Answer from the drawing. Dimensions are ordinates in mm from the lowest x, y and z of the part. A direction names the side the tool comes from. Coordinates: 2 decimals unless noted, no trailing zeros. Loops run counter-clockwise (first coordinate to the right, second up) from the corner with the lowest first, then second, coordinate; pieces in that order, holes last. Notation, with made-up numbers: (-6, 49) -> (47, 49) arc R14 ccw to (47, 57) -> close; hole circle Ø10 at (-20, 82.5). An arc over 180 degrees is marked (long way). Use a Markdown table: item, result.
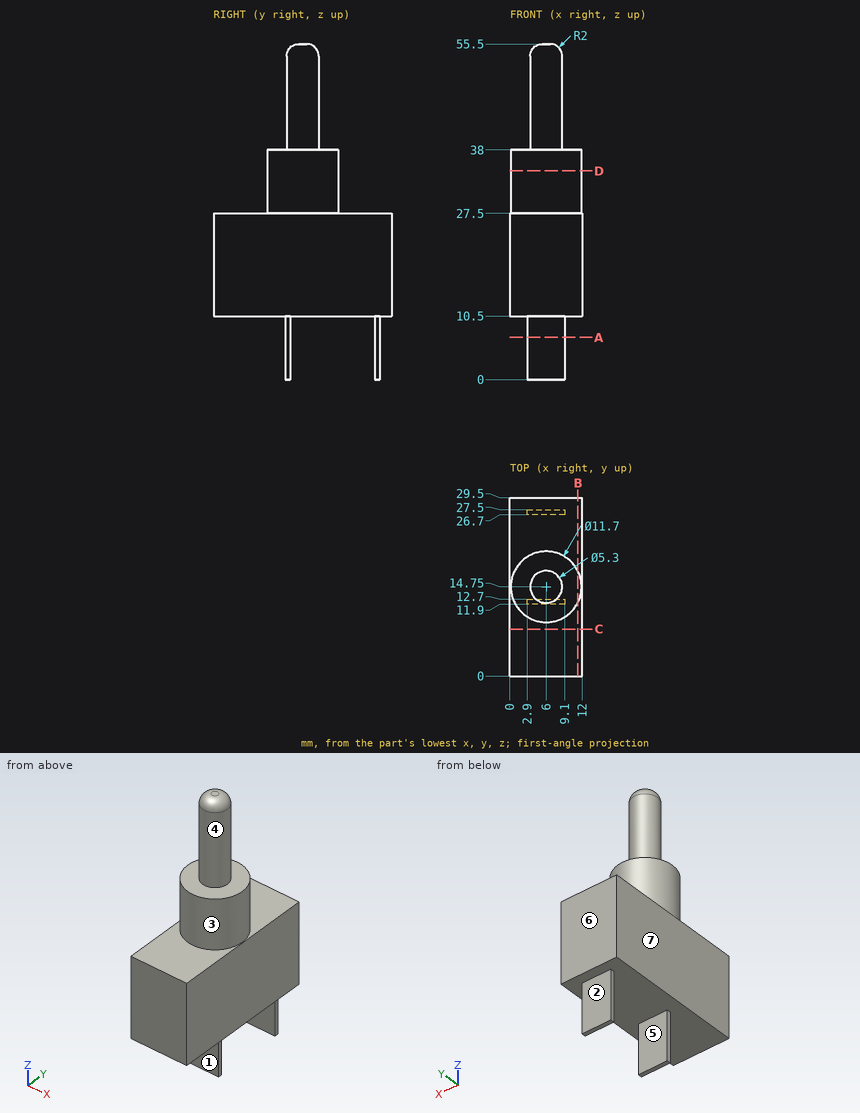
Q1. Consider line 1 (Y direction, x = 8.5, z = 6); line 2 (Z direction, x = 6.5, y = 19.25); line 3 (Z direction, x = 1.5, y = 10). Determine where each line is inside the solid, lowest interval first. Write a range as [from, to].
Solved:
| item | result |
|---|---|
| line 1 | [11.9, 12.7], [26.7, 27.5] |
| line 2 | [10.5, 38] |
| line 3 | [10.5, 27.5] |
Q2. Section B-B on x = 11.25 is taken. Determine the outline of the cut face in (y, z), and give its area (3 significant figures).
Solved:
| item | result |
|---|---|
| outline | (0, 10.5) -> (29.5, 10.5) -> (29.5, 27.5) -> (17.33, 27.5) -> (17.33, 38) -> (12.17, 38) -> (12.17, 27.5) -> (0, 27.5) -> close |
| area | 556 mm² |
Q3. Determine the mould class of the marked faces 4, 5, 6 and 7 for opening direction Y: pulls with the +Y half, pulls with the -Y half, needs draft (parallel to the pull), parting line crosses it, or undercut.
Solved:
| item | result |
|---|---|
| face 4 | parting line crosses it |
| face 5 | undercut |
| face 6 | pulls with the +Y half |
| face 7 | needs draft |
Q4. For the marked faces 1, 2 and 3, determine the directions among +Z, -Z, +X, -X, +Y, -Y from which every point of the face is accessible in a straight line to the end or side of a thin tool.
Solved:
| item | result |
|---|---|
| face 1 | -Z, +X, -X, -Y |
| face 2 | -Z, +X, -X, +Y |
| face 3 | +Z |
Q5. Section C-C on y = 7.75 is taken. Determine the outline of the cut face in (x, z), and give its area (3 significant figures).
Solved:
| item | result |
|---|---|
| outline | (0, 10.5) -> (12, 10.5) -> (12, 27.5) -> (0, 27.5) -> close |
| area | 204 mm² |
Q6. Section A-A on z = 7 is taken. Determine the outline of the cut face in (x, y), and give its area (3 significant figures).
Solved:
| item | result |
|---|---|
| outline | (2.9, 11.9) -> (9.1, 11.9) -> (9.1, 12.7) -> (2.9, 12.7) -> close; (2.9, 26.7) -> (9.1, 26.7) -> (9.1, 27.5) -> (2.9, 27.5) -> close |
| area | 9.92 mm² |
Q7. Given pin 1 Ø5 at (x, z) = (4.5, 7) entering from +Y; pin 2 Ø0.6 at (y, z) = (12.5, 4) entering from -X; pin 3 Ø1 at (x, z) = (9, 30) entering from +Y; pin 4 Ø8 at (y, z) = (23.5, 45) entering from +X, each flat-ended and moving along its own axis, determine where each tip first touches the part or whether it passes through.
Solved:
| item | result |
|---|---|
| pin 1 | y = 27.5 |
| pin 2 | x = 2.9 |
| pin 3 | y = 20.04 |
| pin 4 | through |
Q8. Section D-D on z = 34.5 is taken. Determine the outline of the cut face in (x, y), and give its area (3 significant figures).
Solved:
| item | result |
|---|---|
| outline | circle Ø11.7 at (6, 14.75) |
| area | 108 mm² |
